Here's how the part is built. I have some questions about the finished solid (model axes, mm). A direction names the side the tool comes from. Round coordinates to 2 decimals unless told otherwise and drop trailing zeros. Order: outer loops, then holes, each group sorted by start corner. A loop starts at its lowest first (then second) coordinate and runs counter-clockwise, first axis right, second up. Notation, with made-up numbers: (-29, 62.5) - (-12, 62.5) arc R22 cw to (-12, 70.5) - close; hole circle Ø4 at (64.25, -1). An arc over 180 degrees is marked (long way). Answer as a JSON object with one key per item and string values.
```python
from build123d import *

# Parameters (mm, degrees)
SKETCH1_W           = 127
SKETCH1_H           = 127
SKETCH1_W_2         = 121
SKETCH1_H_2         = 121
SKETCH1_R           = 38.5
BOSS_EXTRUDE1_DEPTH = 13.5
FILLET1_R           = 6.35
SKETCH2_R           = 1.5
CUT_EXTRUDE1_DEPTH  = 91.811618199
BOSS_EXTRUDE2_DEPTH = 100
SKETCH5_R           = 1.5
BOSS_EXTRUDE3_DEPTH = 13.5


with BuildPart() as part:
    # Sketch1 → Boss-Extrude1 (new body)
    with BuildSketch(Plane.XY):
        Rectangle(SKETCH1_W, SKETCH1_H)
        Rectangle(SKETCH1_W_2, SKETCH1_H_2, mode=Mode.SUBTRACT)
        Rectangle(SKETCH1_W_2, SKETCH1_H_2)
        Circle(SKETCH1_R, mode=Mode.SUBTRACT)
        Circle(SKETCH1_R)
    extrude(amount=BOSS_EXTRUDE1_DEPTH)

    # Fillet1
    fillet1_edges = [part.edges().sort_by_distance(p)[0] for p in [
        (-63.5, 63.5, 6.75),
        (63.5, 63.5, 6.75),
        (63.5, -63.5, 6.75),
        (-63.5, -63.5, 6.75),
    ]]
    fillet(fillet1_edges, radius=FILLET1_R)

    # Sketch2 → Cut-Extrude1 (cut, through all)
    with BuildSketch(Plane.XY.offset(13.5)):
        with Locations(Location((57.15, 57.15, 0), (0, 0, 180))):
            Circle(SKETCH2_R)
        with Locations((57.15, -57.15)):
            Circle(SKETCH2_R)
        with Locations((-57.15, 57.15)):
            Circle(SKETCH2_R)
        with Locations(Location((-57.15, -57.15, 0), (0, 0, 180))):
            Circle(SKETCH2_R)
        with BuildLine():
            Line((53.8, 57.15), (53.8, 60.5))
            Line((53.8, 60.5), (-53.8, 60.5))
            Line((-53.8, 60.5), (-53.8, 57.15))
            ThreePointArc((-53.8, 57.15), (-54.781192283, 54.781192283), (-57.15, 53.8))
            Line((-57.15, 53.8), (-60.5, 53.8))
            Line((-60.5, 53.8), (-60.5, -53.8))
            Line((-60.5, -53.8), (-57.15, -53.8))
            ThreePointArc((-57.15, -53.8), (-54.781192283, -54.781192283), (-53.8, -57.15))
            Line((-53.8, -57.15), (-53.8, -60.5))
            Line((-53.8, -60.5), (53.8, -60.5))
            Line((53.8, -60.5), (53.8, -57.15))
            ThreePointArc((53.8, -57.15), (54.781192283, -54.781192283), (57.15, -53.8))
            Line((57.15, -53.8), (60.5, -53.8))
            Line((60.5, -53.8), (60.5, 53.8))
            Line((60.5, 53.8), (57.15, 53.8))
            ThreePointArc((57.15, 53.8), (54.781192283, 54.781192283), (53.8, 57.15))
        make_face()
    extrude(amount=-CUT_EXTRUDE1_DEPTH, mode=Mode.SUBTRACT)

    # Sketch4 → Boss-Extrude2 (add)
    with BuildSketch(Plane(origin=(0, 0, 0), x_dir=(-1, 0, 0), z_dir=(0, 0, -1))):
        with BuildLine():
            ThreePointArc((63.5, 57.15), (61.640128061, 61.640128061), (57.15, 63.5))
            Line((57.15, 63.5), (-57.15, 63.5))
            ThreePointArc((-57.15, 63.5), (-61.640128061, 61.640128061), (-63.5, 57.15))
            Line((-63.5, 57.15), (-63.5, -57.15))
            ThreePointArc((-63.5, -57.15), (-61.640128061, -61.640128061), (-57.15, -63.5))
            Line((-57.15, -63.5), (57.15, -63.5))
            ThreePointArc((57.15, -63.5), (61.640128061, -61.640128061), (63.5, -57.15))
            Line((63.5, -57.15), (63.5, 57.15))
        make_face()
        with BuildLine():
            Line((53.8, 60.5), (57.15, 60.5))
            ThreePointArc((57.15, 60.5), (59.518807717, 59.518807717), (60.5, 57.15))
            Line((60.5, 57.15), (60.5, 53.8))
            Line((60.5, 53.8), (60.5, -53.8))
            Line((60.5, -53.8), (60.5, -57.15))
            ThreePointArc((60.5, -57.15), (59.518807717, -59.518807717), (57.15, -60.5))
            Line((57.15, -60.5), (53.8, -60.5))
            Line((53.8, -60.5), (-53.8, -60.5))
            Line((-53.8, -60.5), (-57.15, -60.5))
            ThreePointArc((-57.15, -60.5), (-59.518807717, -59.518807717), (-60.5, -57.15))
            Line((-60.5, -57.15), (-60.5, -53.8))
            Line((-60.5, -53.8), (-60.5, 53.8))
            Line((-60.5, 53.8), (-60.5, 57.15))
            ThreePointArc((-60.5, 57.15), (-59.518807717, 59.518807717), (-57.15, 60.5))
            Line((-57.15, 60.5), (-53.8, 60.5))
            Line((-53.8, 60.5), (53.8, 60.5))
        make_face(mode=Mode.SUBTRACT)
    extrude(amount=BOSS_EXTRUDE2_DEPTH)

    # Sketch5 → Boss-Extrude3 (add)
    with BuildSketch(Plane(origin=(0, 0, -100), x_dir=(-1, 0, 0), z_dir=(0, 0, -1))):
        with BuildLine():
            Line((63.5, -57.15), (63.5, 57.15))
            ThreePointArc((63.5, 57.15), (61.640128061, 61.640128061), (57.15, 63.5))
            Line((57.15, 63.5), (-57.15, 63.5))
            ThreePointArc((-57.15, 63.5), (-61.640128061, 61.640128061), (-63.5, 57.15))
            Line((-63.5, 57.15), (-63.5, -57.15))
            ThreePointArc((-63.5, -57.15), (-61.640128061, -61.640128061), (-57.15, -63.5))
            Line((-57.15, -63.5), (57.15, -63.5))
            ThreePointArc((57.15, -63.5), (61.640128061, -61.640128061), (63.5, -57.15))
        make_face()
        with BuildLine():
            Line((-60.5, -57.15), (-60.5, 57.15))
            ThreePointArc((-60.5, 57.15), (-59.518807717, 59.518807717), (-57.15, 60.5))
            Line((-57.15, 60.5), (57.15, 60.5))
            ThreePointArc((57.15, 60.5), (59.518807717, 59.518807717), (60.5, 57.15))
            Line((60.5, 57.15), (60.5, -57.15))
            ThreePointArc((60.5, -57.15), (59.518807717, -59.518807717), (57.15, -60.5))
            Line((57.15, -60.5), (-57.15, -60.5))
            ThreePointArc((-57.15, -60.5), (-59.518807717, -59.518807717), (-60.5, -57.15))
        make_face(mode=Mode.SUBTRACT)
        with BuildLine():
            Line((-57.15, -53.8), (-60.5, -53.8))
            Line((-60.5, -53.8), (-60.5, -57.15))
            ThreePointArc((-60.5, -57.15), (-59.518807717, -59.518807717), (-57.15, -60.5))
            Line((-57.15, -60.5), (-53.8, -60.5))
            Line((-53.8, -60.5), (-53.8, -57.15))
            ThreePointArc((-53.8, -57.15), (-54.781192283, -54.781192283), (-57.15, -53.8))
        make_face()
        with Locations(Location((-57.15, -57.15, 0), (0, 0, 180))):
            Circle(SKETCH5_R, mode=Mode.SUBTRACT)
        with BuildLine():
            Line((60.5, -57.15), (60.5, -53.8))
            Line((60.5, -53.8), (57.15, -53.8))
            ThreePointArc((57.15, -53.8), (54.781192283, -54.781192283), (53.8, -57.15))
            Line((53.8, -57.15), (53.8, -60.5))
            Line((53.8, -60.5), (57.15, -60.5))
            ThreePointArc((57.15, -60.5), (59.518807717, -59.518807717), (60.5, -57.15))
        make_face()
        with Locations((57.15, -57.15)):
            Circle(SKETCH5_R, mode=Mode.SUBTRACT)
        with BuildLine():
            Line((57.15, 60.5), (53.8, 60.5))
            Line((53.8, 60.5), (53.8, 57.15))
            ThreePointArc((53.8, 57.15), (54.781192283, 54.781192283), (57.15, 53.8))
            Line((57.15, 53.8), (60.5, 53.8))
            Line((60.5, 53.8), (60.5, 57.15))
            ThreePointArc((60.5, 57.15), (59.518807717, 59.518807717), (57.15, 60.5))
        make_face()
        with Locations(Location((57.15, 57.15, 0), (0, 0, 180))):
            Circle(SKETCH5_R, mode=Mode.SUBTRACT)
        with BuildLine():
            Line((-53.8, 57.15), (-53.8, 60.5))
            Line((-53.8, 60.5), (-57.15, 60.5))
            ThreePointArc((-57.15, 60.5), (-59.518807717, 59.518807717), (-60.5, 57.15))
            Line((-60.5, 57.15), (-60.5, 53.8))
            Line((-60.5, 53.8), (-57.15, 53.8))
            ThreePointArc((-57.15, 53.8), (-54.781192283, 54.781192283), (-53.8, 57.15))
        make_face()
        with Locations((-57.15, 57.15)):
            Circle(SKETCH5_R, mode=Mode.SUBTRACT)
    extrude(amount=BOSS_EXTRUDE3_DEPTH)


solid = part.part
```
1. For faces 1 (the face through (-54.755, 54.807, -106.656)), 2 (the face through (59, 57, -100)), 3 (the face through (1, -63.5, -49)), which set-ups out of +Z, -Z, +X, -X, +Y, -Y let a thin tool reach every point of the face, with its end or its side?
Responses:
{"face 1": "+Z, -Z", "face 2": "none", "face 3": "+Z, -Z, +X, -X, -Y"}
2. Imagine slicing it at A-A (y = -40). List the corners of the cut face in (x, z) for me.
Responses:
{"outline": "(-63.5, -113.5) - (-60.5, -113.5) - (-60.5, 13.5) - (-63.5, 13.5) - close; (60.5, -113.5) - (63.5, -113.5) - (63.5, 13.5) - (60.5, 13.5) - close"}
3. Thinking about a two-plate mould opening in Z: for faces 4 (the face through (53.8, -59, -107)), 5 (the face through (-59, 57, 0)), 6 (the face through (59.493, -59.545, -49.3)), 7 (the face through (5, -61, -113.5)), which applies, pulls with the +Z half, pulls with the -Z half, needs draft (parallel to the pull), parting line crosses it, or undercut?
Responses:
{"face 4": "needs draft", "face 5": "undercut", "face 6": "undercut", "face 7": "pulls with the -Z half"}
4. For P1, Ø3.5, axis at x = 57.15, y = -57.15, coming from the +Z side; P2, Ø1, axis at y = -59.5, z = 8, coming from the +X side; P3, Ø1.7, axis at y = 59, z = 7.5, coming from the +X side; P4, Ø1, axis at y = -58, z = 6.5, coming from the -X side, each with a flat end and sliding along its axis, tell me the tip position at first contact or that it passes through.
Responses:
{"P1": "z = 13.5", "P2": "x = 63.22", "P3": "x = 63.42", "P4": "x = -63.49"}
5. If I drill on L1, parallel to Y at x = 57.15, z = -104.5; L2, parallel to X at y = -57, z = -104; L3, parallel to Y at x = 8, z = 4.5, over which ranges is the centre line in solid material (lowest first)? Write a range as [from, to].
Responses:
{"L1": "[-63.5, -58.65], [-55.65, -53.8], [53.8, 55.65], [58.65, 63.5]", "L2": "[-63.5, -58.64], [-55.66, -53.8], [53.8, 55.66], [58.64, 63.5]", "L3": "[-63.5, -60.5], [60.5, 63.5]"}
6. Imagine slicing it at B-B (z = -66). List the corners of the cut face in (x, y) for me.
Responses:
{"outline": "(-63.5, -57.15) arc R6.35 ccw to (-57.15, -63.5) - (57.15, -63.5) arc R6.35 ccw to (63.5, -57.15) - (63.5, 57.15) arc R6.35 ccw to (57.15, 63.5) - (-57.15, 63.5) arc R6.35 ccw to (-63.5, 57.15) - close; hole (-60.5, -57.15) arc R3.35 ccw to (-57.15, -60.5) - (57.15, -60.5) arc R3.35 ccw to (60.5, -57.15) - (60.5, 57.15) arc R3.35 ccw to (57.15, 60.5) - (-57.15, 60.5) arc R3.35 ccw to (-60.5, 57.15) - close"}
